from build123d import *

# Parameters (mm, degrees)
PAD_DEPTH       = 40
SKETCH001_W     = 12
SKETCH001_H     = 11
SKETCH001_R     = 1.6
PAD001_DEPTH    = 2
SKETCH002_R     = 1.6
PAD002_DEPTH    = 1
POCKET_DEPTH    = 20.001
PAD003_DEPTH    = 34
SKETCH005_R     = 3
POCKET001_DEPTH = 11
SKETCH006_R     = 1.55
POCKET002_DEPTH = 5


with BuildPart() as part:
    # Sketch → Pad (new body)
    with BuildSketch(Plane.YZ):
        with BuildLine():
            Line((-5, 8), (-5, 9))
            Line((-5, 9), (-6, 9))
            Line((-6, 9), (-6, -2))
            Line((-6, -2), (6, -2))
            Line((6, -2), (6, 9))
            Line((6, 9), (5, 9))
            Line((5, 9), (5, 8))
            ThreePointArc((5, 8), (3.556624, 5.5), (5, 3))
            Line((5, 3), (5, 0))
            Line((5, 0), (2.5, 0))
            ThreePointArc((2.5, 0), (0, 1.443376), (-2.5, 0))
            Line((-2.5, 0), (-5, 0))
            Line((-5, 0), (-5, 3))
            ThreePointArc((-5, 3), (-3.556624, 5.5), (-5, 8))
        make_face()
    extrude(amount=PAD_DEPTH)

    # Sketch001 (on Face15 of Pad) → Pad001 (join)
    with BuildSketch(Plane(origin=(0, 0, 0), x_dir=(0, 1, 0), z_dir=(-1, 0, 0))):
        with Locations((0, -3.5)):
            Rectangle(SKETCH001_W, SKETCH001_H)
        with Locations((0, -5)):
            Circle(SKETCH001_R, mode=Mode.SUBTRACT)
    extrude(amount=PAD001_DEPTH)

    # Sketch002 (on Face16 of Pad001) → Pad002 (join, symmetric)
    with BuildSketch(Plane.YX.offset(2)):
        with BuildLine():
            Line((-10, 29), (10, 29))
            ThreePointArc((14, 25), (12.828427, 27.828427), (10, 29))
            Line((14, 25), (14, 15))
            ThreePointArc((10, 11), (12.828427, 12.171573), (14, 15))
            Line((10, 11), (-10, 11))
            ThreePointArc((-14, 15), (-12.828427, 12.171573), (-10, 11))
            Line((-14, 15), (-14, 25))
            ThreePointArc((-10, 29), (-12.828427, 27.828427), (-14, 25))
        make_face()
        with Locations((-10, 25)):
            Circle(SKETCH002_R, mode=Mode.SUBTRACT)
        with Locations((-10, 15)):
            Circle(SKETCH002_R, mode=Mode.SUBTRACT)
        with Locations((10, 15)):
            Circle(SKETCH002_R, mode=Mode.SUBTRACT)
        with Locations((10, 25)):
            Circle(SKETCH002_R, mode=Mode.SUBTRACT)
    extrude(amount=PAD002_DEPTH, both=True)

    # Sketch003 (on Face7 of Pad002) → Pocket (cut, through all)
    with BuildSketch(Plane(origin=(0, -6, 0), x_dir=(0, 0, -1), z_dir=(0, -1, 0))):
        with BuildLine():
            Line((-9, 0.4), (-4.5, 0.4))
            ThreePointArc((-4.5, 0.4), (-3.085786, 0.985786), (-2.5, 2.4))
            Line((-2.5, 2.4), (-2.5, 5.4))
            Line((-2.5, 5.4), (-9, 5.4))
            Line((-9, 5.4), (-9, 0.4))
        make_face()
    extrude(amount=-POCKET_DEPTH, mode=Mode.SUBTRACT)

    # Sketch004 (on Face23 of Pocket) → Pad003 (join)
    with BuildSketch(Plane.YZ.offset(40)):
        Polygon((-6, 9), (-10, -2), (10, -2), (6, 9), (6, -1), (-6, -1), align=None)
    extrude(amount=-PAD003_DEPTH)

    # Sketch005 (on Face52 of Pad003) → Pocket001 (cut)
    with BuildSketch(Plane(origin=(0, 0, -1), x_dir=(0, -1, 0), z_dir=(0, 0, 1))):
        with Locations((-10, 25)):
            Circle(SKETCH005_R)
        with Locations((10, 25)):
            Circle(SKETCH005_R)
        with Locations((10, 15)):
            Circle(SKETCH005_R)
        with Locations((-10, 15)):
            Circle(SKETCH005_R)
    extrude(amount=POCKET001_DEPTH, mode=Mode.SUBTRACT)

    # Sketch006 (on Face52 of Pocket001) → Pocket002 (cut)
    with BuildSketch(Plane(origin=(0, 0, -1), x_dir=(0, -1, 0), z_dir=(0, 0, 1))):
        with Locations((-10, 25)):
            Circle(SKETCH006_R)
        with Locations((-10, 15)):
            Circle(SKETCH006_R)
        with Locations((10, 25)):
            Circle(SKETCH006_R)
        with Locations((10, 15)):
            Circle(SKETCH006_R)
    extrude(amount=-POCKET002_DEPTH, mode=Mode.SUBTRACT)


solid = part.part
Input: part model. Units: mm. Frame: model coordinates. A direction names the side the tool comes from. Give positions to 0.01 mm unless a question says otherwise; leave off trailing zeros. Loops run counter-clockwise (first coordinate to the right, second up) from the corner with the lowest first, then second, coordinate; pieces in that order, holes last. Notation, with made-up numbers: (78, -39.5) -> (121, -39.5) arc R19 ccw to (121, -35.5) -> close; hole circle Ø9 at (-27.5, 8). An arc over 180 degrees is marked (long way). Answer as a JSON object with one key per item and string values. Group by question number.
Item 1: Cut plane A-A, the plane y = 0. Return the cut outline in (x, z), and give its area (3 significant figures).
Item 2: Pull-direction query (Y, two-part tool) for faces 4 (the flat face through (3.9, 5.5, 2.5)), 5 (the flat face through (20, 5, 2)), 6 (the flat face through (20, 14, -2)); classes: released by +Y, released by -Y, zero draft, split by the parting line, or undercut.
Item 3: Pin query (flat end, axial travel): P1, Ø0.8, axis at x = 24.5, y = -9, coming from the -Z side; P2, Ø0.8, axis at x = 3.5, y = 5.5, coming from the +Z side; P3, Ø3, axis at x = 11.5, y = -0.5, coming from the +Z side; P4, Ø0.8, axis at x = 20, z = 8.5, coming from the -Y side. Return the tip coordinate at first contact, or that it passes through.
Item 4: Line query: probe 1 along Y at (x, z) = (25, -1.7); probe 2 along Y at (x, z) = (25, -2.5); probe 3 along X at (y, z) = (10, -2.45). Output: solid intervals per line, ascending.
Item 5: Reachability of faces 1 (the flat face through (2, -6, 2)), 2 (the cylindrical face through (0.75, -5.14, 3.37)), 3 (the cylindrical face through (14.97, 8.45, -1.49)) from +Z, -Z, +X, -X, +Y, -Y: full face, straight path, thin tool, end or side. Return the list, or none.
Item 6: Cut plane C-C, the plane y = -6.5. Return the cut outline in (x, z) (3 decimals).
Item 7: Cut plane B-B, the plane z = 5. State how many separate pieces and enclosed holes the cut face has, and give its area (3 significant figures).
Checks:
{
 "1": {"outline": "(-2, -2) -> (11, -2) -> (11, -3) -> (29, -3) -> (29, -2) -> (40, -2) -> (40, 1.44) -> (0, 1.44) -> (0, 3.4) -> (-2, 3.4) -> close; (-2, 6.6) -> (0, 6.6) -> (0, 9) -> (-2, 9) -> close", "area": "171 mm²"},
 "2": {"face 4": "zero draft", "face 5": "undercut", "face 6": "released by +Y"},
 "3": {"P1": "passes through", "P2": "stops at z = 2.5", "P3": "stops at z = 1.44", "P4": "stops at y = -6.33"},
 "4": {"probe 1": "y = -14 to -11.6, -8.45 to 8.45, 11.6 to 14", "probe 2": "y = -14 to -11.6, -8.4 to 8.4, 11.6 to 14", "probe 3": "x = 11 to 13.4, 16.6 to 23.4, 26.6 to 29"},
 "5": {"face 1": "+Z, -Z, -X, -Y", "face 2": "+Z, +Y, -Y", "face 3": "+Z, -Z"},
 "6": {"outline": "(6, -2) -> (11, -2) -> (11, -3) -> (29, -3) -> (29, -2) -> (40, -2) -> (40, 7.625) -> (6, 7.625) -> close"},
 "7": {"separate pieces": "4", "enclosed holes": "0", "area": "281 mm²"}
}
